Autodesk Inventor part; units mm, degrees
ref_plane "Start Plane" through (0, 0, -12.7) normal (0, 0, 1) x (1, 0, 0)
ref_plane "End Plane" through (0, 0, 1012.7) normal (0, 0, 1) x (1, 0, 0)
ref_plane "Work Plane4" through (12.7, 0, 1012.7) normal (0, 0.7071, 0.7071) x (1, 0, 0)
ref_plane "Start Plane" through (0, 0, -12.7) normal (0, 0, 1) x (1, 0, 0)
ref_plane "End Plane" through (0, 0, 1012.7) normal (0, 0, 1) x (1, 0, 0)
sketch "Sketch" plane through (0, 0, 0) normal (0, 0, 1) x (1, 0, 0)
  line L0 (25.4, 0) -> (0, 0)
  line L1 (0, 0) -> (0, 25.4)
  line L2 (0, 25.4) -> (1.651, 25.4)
  line L3 (3.175, 23.876) -> (3.175, 6.477)
  line L4 (6.477, 3.175) -> (23.876, 3.175)
  line L5 (25.4, 1.651) -> (25.4, 0)
  line L6 (0, -11.0414) -> (0, 31.5385) construction
  line L7 (-11.0414, 0) -> (31.5385, 0) construction
  arc A0 (3.175, 6.477) -> (6.477, 3.175) centre (6.477, 6.477) ccw
  arc A1 (3.175, 23.876) -> (1.651, 25.4) centre (1.651, 23.876) ccw
  arc A2 (25.4, 1.651) -> (23.876, 3.175) centre (23.876, 1.651) ccw
  line L8 (0, 40.0545) -> (0, -19.5574) construction
  line L9 (-19.5574, 0) -> (40.0545, 0) construction
  point P0 (3.175, 25.4)
  point P1 (3.175, 3.175)
  point P2 (25.4, 3.175)
  dimension "d0" = 25.4
  dimension "d1" = 25.4
  dimension "d2" = 3.175
  dimension "d3" = 3.175
  dimension "d10" = 0
  dimension "d11" = 0
  dimension "d14" = 3.302
  dimension "d15" = 1.524
extrude "Body" add sketch "Sketch" along normal up to surface (1025.4 mm away) from surface at -12.7
sketch "Sketch3" plane through (0, 0, 0) normal (0, 0, 1) x (1, 0, 0)
  line L0 (0, 0) -> (10, 0)
ref_plane "Work Plane3" through (0, 0, 0) normal (0, -1, 0) x (1, 0, 0)
ref_plane "Work Plane4" through (12.7, 0, 1012.7) normal (0, 0.7071, 0.7071) x (1, 0, 0)
split "Split1" plane through (12.7, 0, 1012.7) removes the side toward (0, 0.7071, 0.7071)
ref_plane "Work Plane5" through (12.7, 0, -12.7) normal (0, 0.7071, -0.7071) x (1, 0, 0)
split "Split2" plane through (12.7, 0, -12.7) removes the side toward (0, 0.7071, -0.7071)
sketch "Sketch4" plane through (0, 0, 0) normal (0, -1, 0) x (1, 0, 0)
  line L0 (-2, -12.7) -> (12, -12.7)
  line L1 (-2, 1012.7) -> (12, 1012.7)
  dimension "d17" = 1025.4
equation "\"d0\" = G_H"
equation "\"d1\" = G_H"
equation "\"d2\" = G_T"
equation "\"d3\" = G_T"
equation "\"d14\" = G_IR"
equation "\"d15\" = G_ER"
equation "\"d4\" = G_L"
equation "\"G_H\" = 25.4"
equation "\"G_T\" = 3.175"
equation "\"G_ER\" = 1.524"
equation "\"G_IR\" = 3.302"
equation "\"G_L\" = d17"
equation "\"ex\" = 0"
equation "\"G_OFFSET_START\" = 12.7"
equation "\"G_OFFSET_END\" = 12.7"
equation "\"d12\" = -G_OFFSET_START"
equation "\"d13\" = G_OFFSET_END + B_L"
properties part number "AISC - L 1 x 1 x 1/8 - 40.37" material "Steel, Mild"
CAD build for the part. Positions are in the model's coordinates, mm. A direction names the side the tool comes from. Round coordinates to 2 decimals unless told otherwise and drop trailing zeros. Write each loop counter-clockwise with the first axis right and the second up, starting at its lowest first coordinate (ties: lowest second). Pieces come first, ordered by that corner, then holes. Notation, with made-up numbers: (67.25, -16) - (115.25, -16) arc R32 ccw to (115.25, 20) - close; hole circle Ø9 at (16.5, 65). An arc over 180 degrees is marked (long way). Write item = value, one per line. Start each with the question number.
Q1. Probe L1, parallel to X at y = 20.75, z = 99 (3 decimals); L2, parallel to Y at x = 2.25, z = 551. List the from-to ranges inside material, lowest first. Write a range as from..to.
Q2. Band-saw the part on A-A (z = 87.5). Give the cut face in (x, y) (3 decimals), then the cut area to 3 significant figures.
Q3. Which spindle directions (+Z, -Z, +X, -X, +Y, -Y) get a long thin tool onto all of the face, cutting with end or side? Do faces 1 (the flat face through (13, 0, 493)), 2 (the flat face through (3.175, 15, 493)). Say none if no direction does.
Q4. Drop flat-ended pins along their axis: pin 1 (1.5 mm diameter, centred on y = 17.5, z = 817.5, fed in from +X) (3 decimals); pin 2 (5 mm diameter, centred on x = 5.5, z = 210, fed in from +Y); pin 3 (5 mm diameter, centred on x = 15.5, z = 373, fed in from +Y) (3 decimals). Give the stop position or say it passes through.
Q5. Band-saw the part on C-C (x = 19.5). Give the cut face in (y, z) (3 decimals).
Q6. Band-saw the part on B-B (y = 10.75). Give the cut face in (x, z) (3 decimals), then the cut area to 3 significant figures.
Answers below:
q1.L1 = 0..3.175
q1.L2 = 0..25.28
q2.outline = (0, 0) - (25.4, 0) - (25.4, 1.651) arc R1.524 ccw to (23.876, 3.175) - (6.477, 3.175) arc R3.302 cw to (3.175, 6.477) - (3.175, 23.876) arc R1.524 ccw to (1.651, 25.4) - (0, 25.4) - close
q2.area = 153 mm2
q3.face_1 = +Z, -Z, +X, -X, -Y
q3.face_2 = +Z, -Z, +X, +Y
q4.pin_1 = 3.175
q4.pin_2 = 24.59
q4.pin_3 = 3.175
q5.outline = (0, -12.7) - (3.175, -9.525) - (3.175, 1009.525) - (0, 1012.7) - close
q6.outline = (0, -1.95) - (3.175, -1.95) - (3.175, 1001.95) - (0, 1001.95) - close
q6.area = 3,190 mm2
